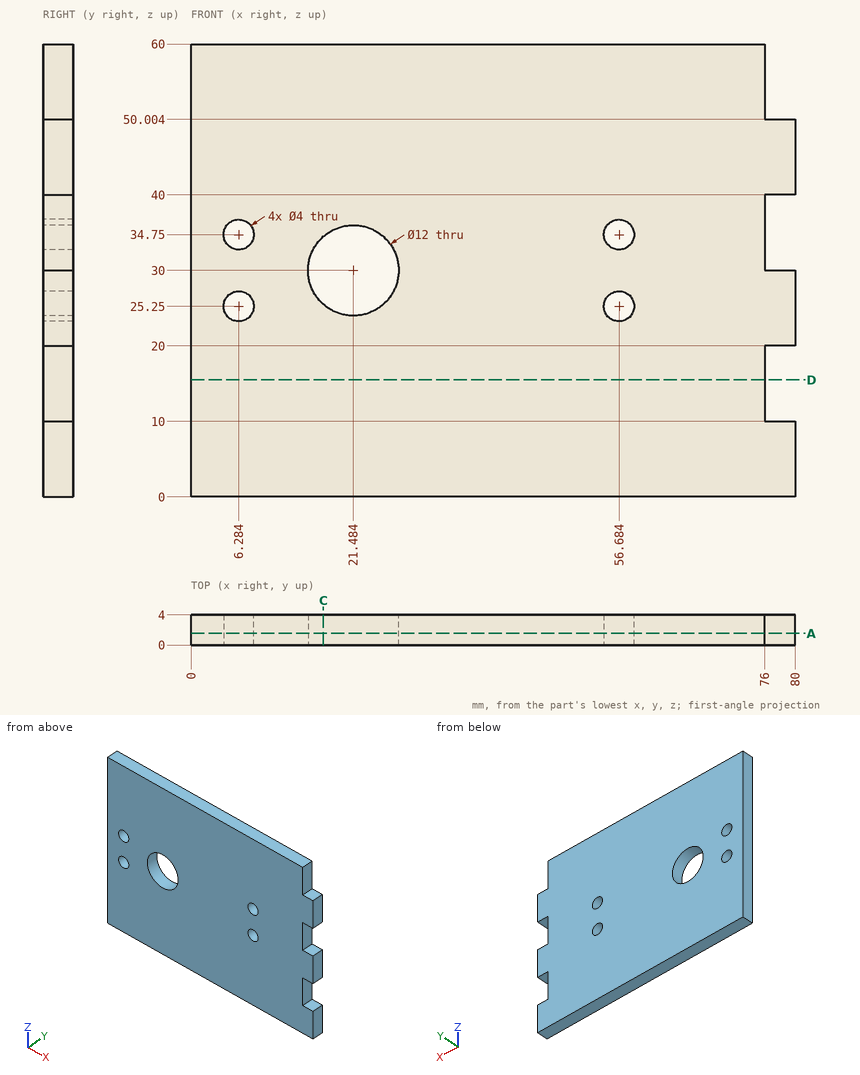
Job drawing, mm, ordinate dimensions from the low corner. One solid piece. Give positions to 0.01 mm unless a question says otherwise; leave off trailing zeros. Order: outer loops, then holes, each group sorted by start corner. A loop starts at its lowest first (then second) coordinate and runs counter-clockwise, first axis right, second up. Notation, with made-up numbers: (30.5, 30) -> (34.5, 30) arc R23 cw to (34.5, 50) -> close; hole circle Ø10 at (69, 77.5). An arc over 180 degrees is marked (long way). Return JSON: item names as keys, results as strings.
Q1. Saw through at A-A (y = 1.55). Count the separate pieces of the cut face and the enclosed holes in it, then the cut area to 3 significant figures.
Working result:
{"separate pieces": "1", "enclosed holes": "5", "area": "4,520 mm²"}
Q2. Flat gauge pins, fed straight in: pin 1 (1.2 mm diameter, centred on y = 2, z = 13, fed in from +X); pin 2 (2.5 mm diameter, centred on x = 6.28, z = 34.75, fed in from +Y). Where does each tip first touch, or does it go through?
Working result:
{"pin 1": "x = 76", "pin 2": "through"}
Q3. Saw through at C-C (x = 17.5). Write the cut outline in (y, z), then the cut area to 3 significant figures.
Working result:
{"outline": "(0, 0) -> (4, 0) -> (4, 25.51) -> (0, 25.51) -> close; (0, 34.49) -> (4, 34.49) -> (4, 60) -> (0, 60) -> close", "area": "204 mm²"}
Q4. Saw through at D-D (z = 15.5). Write the cut outline in (x, y), then the cut area to 3 significant figures.
Working result:
{"outline": "(0, 0) -> (76, 0) -> (76, 4) -> (0, 4) -> close", "area": "304 mm²"}
Q5. Drill centre lines: line 1 (X direction, y = 2.5, z = 24.5) (1 decimal); line 2 (Z direction, x = 5, y = 0.65) (1 decimal); line 3 (Z direction, x = 56, y = 3.85). Where is each one in solid material? Low to high.
Working result:
{"line 1": "0 to 4.4, 8.1 to 19.1, 23.9 to 54.8, 58.5 to 80", "line 2": "0 to 23.7, 26.8 to 33.2, 36.3 to 60", "line 3": "0 to 23.37, 27.13 to 32.87, 36.63 to 60"}
